Build history of the part. All positions in model axes, mm. A direction names the side the tool comes from. Round coordinates to 2 decimals unless told otherwise and drop trailing zeros. Write each loop counter-clockwise with the first axis right and the second up, starting at its lowest first coordinate (ties: lowest second). Pieces come first, ordered by that corner, then holes. Notation, with made-up numbers: M 83.25,72.5 L 130.25,72.5 A10 cw 130.25,85.5 Z; hole C 84.5,-26 d1. An arc over 180 degrees is marked long. Use a Markdown table: item, result.
from build123d import *

# Parameters (mm, degrees)
F0_R           = 8.875
F0_R_2         = 5.875
F1_DEPTH       = 70
F2_START       = 44
F2_DEPTH       = 24
F4_D           = 3
F4_DEPTH       = 10
F4_CSINK_D     = 5
F4_CSINK_ANGLE = 80
F4_TIP         = 0.9012909285


with BuildPart() as f1:
    # F0 (on Right) → F1 (new body)
    with BuildSketch(Plane.YZ):
        Circle(F0_R)
        Circle(F0_R_2, mode=Mode.SUBTRACT)
    extrude(amount=F1_DEPTH)

    # F0 (on Right) → F2 (join)
    with BuildSketch(Plane.YZ.offset(F2_START)):
        Circle(F0_R_2)
    extrude(amount=F2_DEPTH)

    # F4
    with Locations(Plane.YZ.offset(68)):
        with Locations((0, 0)):
            CounterSinkHole(F4_D / 2, F4_CSINK_D / 2, depth=F4_DEPTH, counter_sink_angle=F4_CSINK_ANGLE)
            with Locations((0, 0, -(F4_DEPTH + F4_TIP / 2))):  # 118° drill point
                Cone(0, F4_D / 2, F4_TIP, mode=Mode.SUBTRACT)


solid = f1.part
Q1. Cut at B-B on x = 19.5. Give the cut face in (y, z) (3 decimals).
Response values:
| item | result |
|---|---|
| outline | C 0,0 d17.75; hole C 0,0 d11.75 |
Q2. Cut at D-D on z = 7.25. Give the cut face in (x, y), and give its area (3 significant figures).
Response values:
| item | result |
|---|---|
| outline | M 0,-5.12 L 70,-5.12 L 70,5.12 L 0,5.12 Z |
| area | 717 mm2 |
Q3. Two-plate mould, pull along Z, no slides. Class faces 4 (the cylindrical face through (34.51, -1.924, -8.664)), 5 (the flat face through (0, 2, -6)), 6 (the flat face through (68, 3, 0)): +Z half, -Z half, draft (parallel to the pull), parting line (faces both ways), or undercut.
Response values:
| item | result |
|---|---|
| face 4 | parting line |
| face 5 | draft |
| face 6 | undercut |
Q4. Which spindle directions (+Z, -Z, +X, -X, +Y, -Y) get a long thin tool onto all of the face, cutting with end or side? Do faces 1 (the flat face through (70, 2, -6)), 2 (the cylindrical face through (68.986, 5.604, 1.765)), 3 (the flat face through (44, 0, 0)). Say none if no direction does.
Response values:
| item | result |
|---|---|
| face 1 | +Z, -Z, +X, +Y, -Y |
| face 2 | +X |
| face 3 | -X |
Q5. Cut at A-A on z = 3.25. Give the cut face in (x, y).
Response values:
| item | result |
|---|---|
| outline | M 0,-8.26 L 70,-8.26 L 70,-4.89 L 68,-4.89 L 68,4.89 L 70,4.89 L 70,8.26 L 0,8.26 L 0,4.89 L 44,4.89 L 44,-4.89 L 0,-4.89 Z |
Q6. Drill centre lines: L1, parallel to Z at x = 69.45, y = 0 (3 decimals); L2, parallel to Z at x = 63.25, y = 0 (3 decimals); L3, parallel to X at y = -2.5, z = -4.75. Where is each one in solid material? Low to high.
Response values:
| item | result |
|---|---|
| L1 | z = -8.875 to -5.875, 5.875 to 8.875 |
| L2 | z = -8.875 to -1.5, 1.5 to 8.875 |
| L3 | x = 44 to 68 |
Q7. Drop flat-ended pins along their axis: P1, Ø3.5, axis at y = 0, z = -2.5, coming from the +X side; P2, Ø3.5, axis at y = 0, z = 0, coming from the +X side; P3, Ø2, axis at x = 10.5, z = 2, coming from the -Y side. Give the stop position or say it passes through.
Response values:
| item | result |
|---|---|
| P1 | stops at x = 68 |
| P2 | stops at x = 67.11 |
| P3 | stops at y = -8.82 |
Q8. Cut at C-C on x = 53. Give the cut face in (y, z) (3 decimals).
Response values:
| item | result |
|---|---|
| outline | C 0,0 d17.75 |
